For this review, use the dimensioned drawing (mm, ordinates from the lowest corner) and the shaded views. A direction names the side the tool comes from. Give positions to 0.01 mm unless a question says otherwise; leave off trailing zeros. Order: outer loops, then holes, each group sorted by start corner. A loop starts at its lowest first (then second) coordinate and runs counter-clockwise, first axis right, second up. Notation, with made-up numbers: (21.25, -15.5) - (70.25, -15.5) arc R3 cw to (70.25, -11.5) - close; hole circle Ø5 at (71, 3.5). An arc over 180 degrees is marked (long way). One line per item, written item: value.
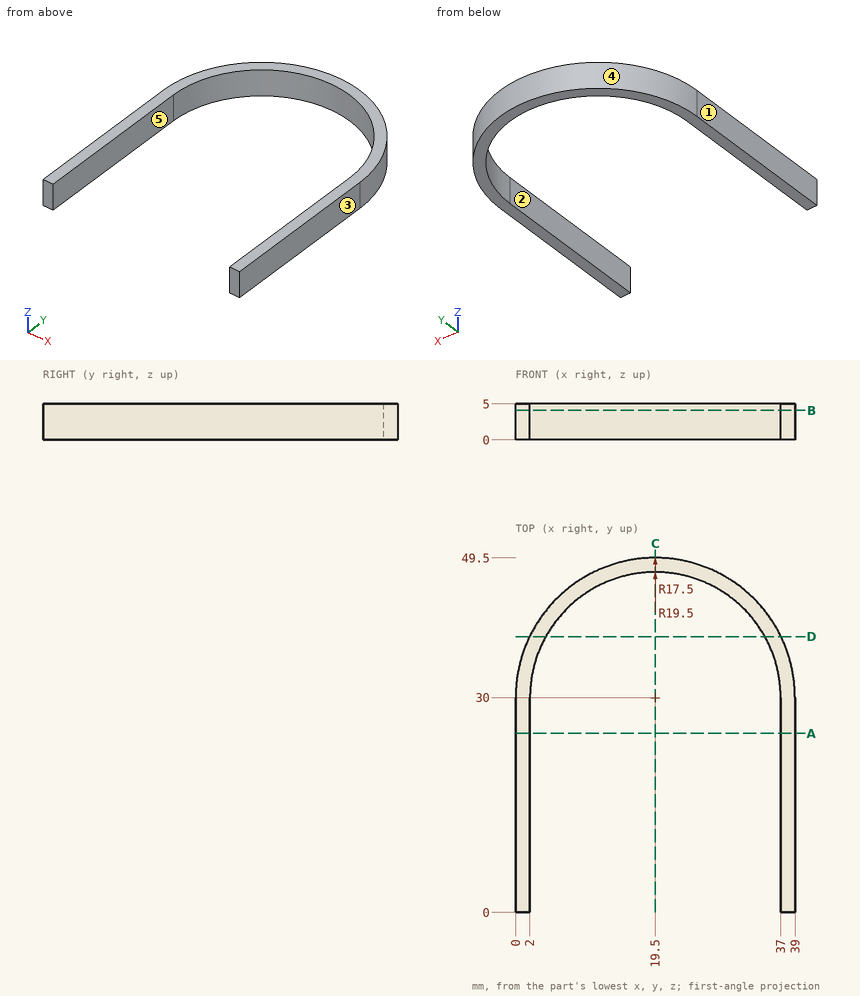
(1) Take a section at D-D (y = 38.5). Write out the cut boundary in (x, z), then the cut area to 3 significant figures.
Answers below:
outline: (1.95, 0) - (4.2, 0) - (4.2, 5) - (1.95, 5) - close; (34.8, 0) - (37.05, 0) - (37.05, 5) - (34.8, 5) - close
area: 22.5 mm^2
(2) Take a section at A-A (y = 25). Write out the cut boundary in (x, z).
Answers below:
outline: (0, 0) - (2, 0) - (2, 5) - (0, 5) - close; (37, 0) - (39, 0) - (39, 5) - (37, 5) - close
(3) Draft analysis for pull direction X (two halves, no side actions). For the marked faces 1, 2 and 3, state which applies: pulls with the +X half, pulls with the -X half, needs draft (parallel to the pull), parting line crosses it, or undercut.
Answers below:
face 1: pulls with the -X half
face 2: undercut
face 3: pulls with the +X half
(4) Take a section at C-C (x = 19.5). Write out the cut boundary in (y, z).
Answers below:
outline: (47.5, 0) - (49.5, 0) - (49.5, 5) - (47.5, 5) - close
(5) Machinability: for the marked faces 4 and 5, which of the approach directions +Z, -Z, +X, -X, +Y, -Y give a long, thin tool a straight path to every point of the face, cutting with its end or side? Answer none if there is none.
Answers below:
face 4: +Z, -Z, +Y
face 5: +Z, -Z, -Y
(6) Wall thickness on line 1 (X direction, y = 16.5, z = 0.2); line 2 (X direction, y = 31.5, z = 1.85); line 3 (Y direction, x = 34.5, z = 1.5): over which ranges is each line inside the solid? List them lowest first. Write a range as from..to.
Answers below:
line 1: x = 0..2, 37..39
line 2: x = 0.06..2.06, 36.94..38.94
line 3: y = 39.01..42.46
(7) For P1, Ø1, axis at x = 10, z = 2.5, coming from the +Y side, flat-tipped, find the tip position at first contact; note if it passes through.
Answers below:
P1: stops at y = 47.3
(8) Take a section at B-B (z = 4.1). Write out the cut boundary in (x, y).
Answers below:
outline: (0, 0) - (2, 0) - (2, 30) arc R17.5 cw to (37, 30) - (37, 0) - (39, 0) - (39, 30) arc R19.5 ccw to (0, 30) - close
